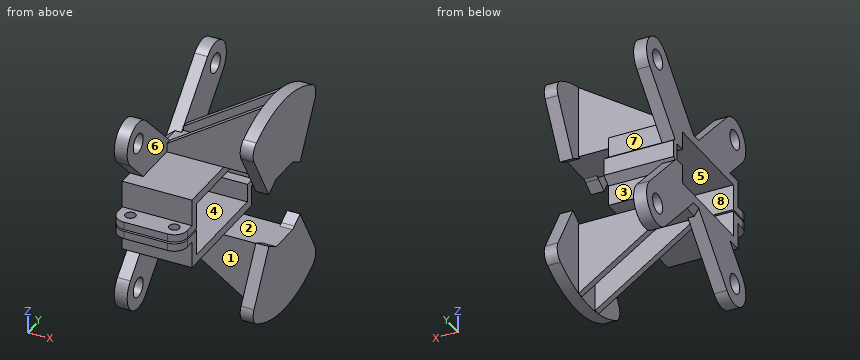
from build123d import *

# Parameters (mm, degrees)
MICRO_START                                  = -46.670460781
MICRO_SERVO_MOUNT_BASE_PART_CAMERA_TUR_DEPTH = 16.1417
MICRO_START_2                                = 12.849763649
MICRO_SERVO_MOUNT_BASE_PART_CAMERA_3_O_R     = 1.2
MICRO_SERVO_MOUNT_BASE_PART_CAMERA_3_DEPTH   = 16.4158
BOSS_EXTRUDE1_DEPTH                          = 4.5
CUT_EXTRUDE1_DEPTH                           = 3
BOSS_EXTRUDE2_DEPTH                          = 3
BOSS_EXTRUDE3_DEPTH                          = 3
FILLET1_R                                    = 3
BOSS_EXTRUDE4_DEPTH                          = 3
CUT_EXTRUDE2_DEPTH                           = 45.721836893
F_8_CLEARANCE_HOLE1_D                        = 4.4958


with BuildPart() as part:
    # Micro Servo Mount Base Part - Camera Tur: read off the stored shape, not the designer's step
    # Micro Servo Mount Base Part - Camera 2 → Micro Servo Mount Base Part - Camera Tur (new body)
    with BuildSketch(Plane.YZ.offset(MICRO_START)):
        Polygon((-18.758887412, 21.257663649), (-11.608887412, 21.257663649), (-11.608887412, 27.265563649), (11.462212588, 27.265563649), (11.462212588, 23.005463649), (13.962212588, 23.005463649), (13.962212588, 19.109863649), (11.462212588, 19.109863649), (11.462212588, 14.849763649), (-11.608887412, 14.849763649), (-11.608887412, 20.857663649), (-18.758887412, 20.857663649), (-18.758887412, 19.057663649), (-13.608887412, 19.057663649), (-13.608887412, 12.849763649), (13.462212588, 12.849763649), (13.462212588, 17.557663649), (15.462212588, 19.057663649), (15.462212588, 23.057663649), (13.462212588, 24.557663649), (13.462212588, 29.265563649), (-13.608887412, 29.265563649), (-13.608887412, 23.057663649), (-18.758887412, 23.057663649), align=None)
    extrude(amount=MICRO_SERVO_MOUNT_BASE_PART_CAMERA_TUR_DEPTH)

    # Micro Servo Mount Base Part - Camera 3 o → Micro Servo Mount Base Part - Camera 3 (cut)
    with BuildSketch(Plane.XY.offset(MICRO_START_2)):
        with BuildLine():
            Line((-46.670460781, -18.758887412), (-43.670460781, -18.758887412))
            ThreePointArc((-43.670460781, -18.758887412), (-45.791781124, -17.880207755), (-46.670460781, -15.758887412))
            Line((-46.670460781, -15.758887412), (-46.670460781, -18.758887412))
        make_face()
        with BuildLine():
            ThreePointArc((-30.528760781, -15.758887412), (-31.407440438, -17.880207755), (-33.528760781, -18.758887412))
            Line((-33.528760781, -18.758887412), (-30.528760781, -18.758887412))
            Line((-30.528760781, -18.758887412), (-30.528760781, -15.758887412))
        make_face()
        with Locations((-43.670460781, -15.758887412)):
            Circle(MICRO_SERVO_MOUNT_BASE_PART_CAMERA_3_O_R)
        with Locations((-33.528760781, -15.758887412)):
            Circle(MICRO_SERVO_MOUNT_BASE_PART_CAMERA_3_O_R)
    extrude(amount=MICRO_SERVO_MOUNT_BASE_PART_CAMERA_3_DEPTH, mode=Mode.SUBTRACT)


with BuildPart() as part_1:
    # Micro Servo Mount Base Part - Camera 4: read off the stored shape, not the designer's step
    # Micro Servo Mount Base Part - Camera 4: moved
    add(part.part.moved(Location((46.6704608, -5.2543126, -21.0576636))))

    # Sketch7 → Boss-Extrude1 (add, symmetric)
    with BuildSketch(Plane(origin=(0, 0, 0), x_dir=(1, 0, 0), z_dir=(0, 1, 0))):
        Polygon((0, 8.2079), (27.8955, 8.2079), (27.8955, 25), (24.8955, 25), align=None)
        Polygon((24.8955, -25), (0, -8.2079), (27.8955, -8.2079), (27.8955, -25), align=None)
    extrude(amount=BOSS_EXTRUDE1_DEPTH, both=True)

    # Sketch9 → Cut-Extrude1 (cut, symmetric)
    with BuildSketch(Plane(origin=(0, 0, 0), x_dir=(1, 0, 0), z_dir=(0, 1, 0))):
        Polygon((1.482572162, -9.2079), (24.8955, -25), (24.8955, -9.2079), align=None)
        Polygon((24.8955, 9.2079), (1.482572162, 9.2079), (24.8955, 25), align=None)
    extrude(amount=CUT_EXTRUDE1_DEPTH, both=True, mode=Mode.SUBTRACT)

    # Sketch10 → Boss-Extrude2 (add)
    with BuildSketch(Plane(origin=(27.8955, 0, 0), x_dir=(0, 0, -1), z_dir=(1, 0, 0))):
        with BuildLine():
            Line((-21.9985795, 12.700885796), (-7.794228634, 4.5))
            ThreePointArc((-7.794228634, 4.5), (-9, 0), (-7.794228634, -4.5))
            Line((-7.794228634, -4.5), (-21.9985795, -12.700885796))
            ThreePointArc((-21.9985795, -12.700885796), (-25.401771592, 0), (-21.9985795, 12.700885796))
        make_face()
        with BuildLine():
            Line((7.794228634, 4.5), (21.9985795, 12.700885796))
            ThreePointArc((21.9985795, 12.700885796), (25.401771592, 0), (21.9985795, -12.700885796))
            Line((21.9985795, -12.700885796), (7.794228634, -4.5))
            ThreePointArc((7.794228634, -4.5), (9, 0), (7.794228634, 4.5))
        make_face()
    extrude(amount=-BOSS_EXTRUDE2_DEPTH)

    # Sketch11 → Boss-Extrude3 (add)
    with BuildSketch(Plane(origin=(27.8955, 0, 0), x_dir=(0, 0, -1), z_dir=(1, 0, 0))):
        Polygon((-21.9985795, 12.700885796), (-7.794228634, 4.5), (-6.294228634, 7.098076211), (-20.4985795, 15.298962007), align=None)
        Polygon((7.794228634, 4.5), (6.294228634, 7.098076211), (20.4985795, 15.298962007), (21.9985795, 12.700885796), align=None)
        Polygon((21.9985795, -12.700885796), (7.794228634, -4.5), (6.294228634, -7.098076211), (20.4985795, -15.298962007), align=None)
        Polygon((-7.794228634, -4.5), (-6.294228634, -7.098076211), (-20.4985795, -15.298962007), (-21.9985795, -12.700885796), align=None)
    extrude(amount=-BOSS_EXTRUDE3_DEPTH)

    # Fillet1
    fillet1_edges = [part_1.edges().sort_by_distance(p)[0] for p in [
        (26.3955, -15.298962007, -20.4985795),
        (26.3955, -15.298962007, 20.4985795),
        (26.3955, 15.298962007, -20.4985795),
        (26.3955, 15.298962007, 20.4985795),
    ]]
    fillet(fillet1_edges, radius=FILLET1_R - 0.0001)  # a hair under: the kernel refuses the full size

    # Sketch13 → Boss-Extrude4 (add)
    with BuildSketch(Plane.ZY):
        with BuildLine():
            Line((13.964466094, -21.035533906), (8.2079, -15.278967812))
            Line((8.2079, -15.278967812), (8.2079, -1.136832188))
            Line((8.2079, -1.136832188), (21.035533906, -13.964466094))
            ThreePointArc((21.035533906, -13.964466094), (21.035533906, -21.035533906), (13.964466094, -21.035533906))
        make_face()
        with BuildLine():
            Line((-13.964466094, 21.035533906), (-1.136832188, 8.2079))
            Line((-1.136832188, 8.2079), (-8.2079, 8.2079))
            Line((-8.2079, 8.2079), (-8.2079, 1.136832188))
            Line((-8.2079, 1.136832188), (-21.035533906, 13.964466094))
            ThreePointArc((-21.035533906, 13.964466094), (-21.035533906, 21.035533906), (-13.964466094, 21.035533906))
        make_face()
        with BuildLine():
            Line((1.136832188, 8.2079), (13.964466094, 21.035533906))
            ThreePointArc((13.964466094, 21.035533906), (21.035533906, 21.035533906), (21.035533906, 13.964466094))
            Line((21.035533906, 13.964466094), (8.2079, 1.136832188))
            Line((8.2079, 1.136832188), (8.2079, 8.2079))
            Line((8.2079, 8.2079), (1.136832188, 8.2079))
        make_face()
        with BuildLine():
            Line((-8.2079, -1.136832188), (-21.035533906, -13.964466094))
            ThreePointArc((-21.035533906, -13.964466094), (-21.035533906, -21.035533906), (-13.964466094, -21.035533906))
            Line((-13.964466094, -21.035533906), (-8.2079, -15.278967812))
            Line((-8.2079, -15.278967812), (-8.2079, -1.136832188))
        make_face()
    extrude(amount=-BOSS_EXTRUDE4_DEPTH)

    # Sketch14 → Cut-Extrude2 (cut, through all)
    with BuildSketch(Plane.ZY):
        Polygon((-1.9478, 6.2079), (-6.2079, 6.2079), (-6.2079, -16.8632), (6.2079, -16.8632), (6.2079, 6.2079), (1.9478, 6.2079), (1.9478, 8.7079), (-1.9478, 8.7079), align=None)
    extrude(amount=-CUT_EXTRUDE2_DEPTH, mode=Mode.SUBTRACT)

    # #8 Clearance Hole1 (through all)
    with Locations(Plane(origin=(3, 0, 0), x_dir=(0, 0, -1), z_dir=(1, 0, 0))):
        with Locations((-17.5, 17.5), (17.5, 17.5), (17.5, -17.5), (-17.5, -17.5)):
            Hole(F_8_CLEARANCE_HOLE1_D / 2)


solid = part_1.part
Check sheet for the modelled part. Datum: model origin and axes. Units: mm. Face numbers are marked on the shaded views. A direction names the side the tool comes from. Round coordinates to 2 decimals unless told otherwise and drop trailing zeros. Order: outer loops, then holes, each group sorted by start corner. A loop starts at its lowest first (then second) coordinate and runs counter-clockwise, first axis right, second up.
(1) Access from +Z, -Z, +X, -X, +Y, -Y to the whole of each face (thin tool, end or side, straight path). Record for the marked faces 1, 2, 3 and 4.
(2) Cross-section at D-D, the plane y = -17.5. Enter the section's corners in (x, z).
(3) Cross-section at A-A, the plane y = -9.5. Enter the section's corners in (x, z).
(4) Cross-section at B-B, the plane x = 18. Enter the section's corners in (y, z), and give its area (3 significant figures).
(5) Cross-section at C-C, the plane z = -19. Enter the section's corners in (x, y), and give its area (3 significant figures).
(6) Scan lines: probe 1 along X at (y, z) = (12, -18); probe 2 along Z at (x, y) = (9.5, -8); probe 3 along Y at (x, z) = (19, 18). Record each from-to range of solid material in increasing order.
(7) Draft check along Y on the marked faces 5, 6, 7 and 8. Enter one of: pulls with the +Y half, pulls with the -Y half, needs draft (parallel to the pull), parting line crosses it, or undercut.
(8) Go/stop test with flat-tipped pins: P1, Ø5, axis at x = 23, y = -12.5, coming from the +Z side; P2, Ø7, axis at x = 7.5, y = -8.5, coming from the +Z side; P3, Ø4.5, axis at x = 5, z = 5, coming from the -Y side; P4, Ø12, axis at y = -2.5, z = 18, coming from the -X side. Record where each tip stops, or that it passes through.
Check sheet entries:
1. face 1: -Z, -Y
1. face 2: none
1. face 3: -Z, +X, +Y
1. face 4: +X, -X
2. outline: (0, -22.5) - (3, -22.5) - (3, -19.75) - (0, -19.75) - close; (0, -15.25) - (3, -15.25) - (3, -10.43) - (0, -10.43) - close; (0, -8.21) - (16.14, -8.21) - (16.14, -0.2) - (0, -0.2) - close; (0, 0.2) - (16.14, 0.2) - (16.14, 8.21) - (0, 8.21) - close; (0, 10.43) - (3, 10.43) - (3, 15.25) - (0, 15.25) - close; (0, 19.75) - (3, 19.75) - (3, 22.5) - (0, 22.5) - close
3. outline: (0, -16.57) - (3, -16.57) - (3, -8.21) - (16.14, -8.21) - (16.14, -6.21) - (0, -6.21) - close; (0, 6.21) - (16.14, 6.21) - (16.14, 8.21) - (3, 8.21) - (3, 16.57) - (0, 16.57) - close; (24.9, -23.56) - (27.9, -23.56) - (27.9, -10.45) - (24.9, -10.45) - close; (24.9, 10.45) - (27.9, 10.45) - (27.9, 23.56) - (24.9, 23.56) - close
4. outline: (-4.5, -20.35) - (-3, -20.35) - (-3, -9.21) - (3, -9.21) - (3, -20.35) - (4.5, -20.35) - (4.5, -8.21) - (-4.5, -8.21) - close; (-4.5, 8.21) - (4.5, 8.21) - (4.5, 20.35) - (3, 20.35) - (3, 9.21) - (-3, 9.21) - (-3, 20.35) - (-4.5, 20.35) - close
4. area: 84.8 mm2
5. outline: (0, -22.27) - (3, -22.27) - (3, -19.17) - (0, -19.17) - close; (0, -15.83) - (3, -15.83) - (3, -11.93) - (0, -11.93) - close; (0, 11.93) - (3, 11.93) - (3, 15.83) - (0, 15.83) - close; (0, 19.17) - (3, 19.17) - (3, 22.27) - (0, 22.27) - close; (16, -4.5) - (24.9, -4.5) - (24.9, -14.17) - (27.9, -14.17) - (27.9, 14.17) - (24.9, 14.17) - (24.9, 4.5) - (16, 4.5) - (16, 3) - (24.9, 3) - (24.9, -3) - (16, -3) - close
5. area: 154 mm2
6. probe 1: x = 0 to 3, 24.9 to 27.9
6. probe 2: z = -8.21 to -6.21, 6.21 to 8.21
6. probe 3: y = -4.5 to -3, 3 to 4.5
7. face 5: undercut
7. face 6: needs draft
7. face 7: pulls with the +Y half
7. face 8: undercut
8. P1: stops at z = 22.96
8. P2: stops at z = 8.21
8. P3: stops at y = -18.86
8. P4: stops at x = 0
